Read the model definition and answer for the solid it produces. Units are mm, in the model's axes. A direction names the side the tool comes from. Coordinates: 2 decimals unless noted, no trailing zeros. Order: outer loops, then holes, each group sorted by start corner. A loop starts at its lowest first (then second) coordinate and runs counter-clockwise, first axis right, second up. Notation, with made-up numbers: (72, 72.25) -> (87, 72.25) arc R19 ccw to (87, 103.25) -> close; hole circle Ø3 at (10, -32.5). An arc over 180 degrees is marked (long way). Answer as a JSON object with one key per item and string values. Group by question number.
1) Section C-C on x = 11 is taken. Determine the outline of the cut face in (y, z) (3 decimals).
2) A tool of negligible diameter and unlimited length cuts with its end or side. For faces 1 (the flat face through (-16.036, 26.611, 7.55)), 2 (the flat face through (10.173, -4.366, 4.696)), 3 (the cylindrical face through (-31.266, 33.461, 4.696)), from which of +Z, -Z, +X, -X, +Y, -Y can it reach the whole face along a straight path? Write none if from no direction.
3) Consider L1, parallel to Z at x = 0, y = 57.7 (3 decimals); L2, parallel to Y at x = 19.5, z = 6.25; L3, parallel to Y at x = 1.5, z = 3.25. Determine where each line is inside the solid, lowest interval first.
4) Given pin 1 (3 mm diameter, centred on x = -0.5, z = 5, fed in from -Y); pin 2 (3 mm diameter, centred on x = 12.5, z = 8.5, fed in from -Y); pin 3 (5 mm diameter, centred on x = 0, y = 13.5, fed in from +Z) (3 decimals), each flat-ended and moving along its own axis, determine where each tip first touches the part or whether it passes through.
5) Determine the mould class of faces 4 (the cylindrical face through (-31.23, -0.04, 4.7)), 5 (the cylindrical face through (6.45, 23.53, 1.25)), 6 (the flat face through (17.07, 54.53, 4.7)) for opening direction X: released by +X, released by -X, zero draft, split by the parting line, or undercut.
6) Section A-A on x = -9.5 is taken. Determine the outline of the cut face in (y, z) (3 decimals), and give its area (3 significant figures).
7) Section B-B on y = 53.5 is taken. Determine the outline of the cut face in (x, z) (1 decimal), and give its area (3 significant figures).
8) Section D-D on y = 7 is taken. Determine the outline of the cut face in (x, z) (3 decimals), and give its area (3 significant figures).
from build123d import *

# Parameters (mm, degrees)
F0_R        = 3.1496
F0_R_2      = 16.51
F1_DEPTH    = 9.525
F0_R_3      = 13.97
F2_DEPTH    = 2.54
F4_DEPTH    = 8.636
F5_T1_DEPTH = 2.54
F5_T3_DEPTH = 2.54
F5_T5_DEPTH = 2.54
F5_T7_DEPTH = 2.54
F5_T9_DEPTH = 2.54
F6_R        = 1.5875
F9_DEPTH    = 5.08
F7_R        = 1.5875
F10_DEPTH   = 20.32
F8_R        = 1.5875
F11_DEPTH   = 20.32
F13_DEPTH   = 2.54


# Not quite as in the source:
# - a fillet or chamfer that OpenCascade refuses, or shapes differently, is made with other operations: its cross-section is extruded or revolved along the edge and cut away or added
# - a feature names something its author has since deleted; it is built from what else it names


with BuildPart() as f1:
    # F0 (on Top) → F1 (new body)
    with BuildSketch(Plane.XY):
        with BuildLine():
            ThreePointArc((6.8331158271, 57.7357942584), (0, 58.780934), (-6.8331158271, 57.7357942584))
            Line((-6.8331158271, 57.7357942584), (-27.0242026981, 51.4112964789))
            ThreePointArc((-27.0242026981, 51.4112964789), (-30.2435047856, 49.1112435687), (-31.4761149683, 45.3516130738))
            Line((-31.4761149683, 45.3516130738), (-31.4761149683, 35.0824113719))
            ThreePointArc((-31.4761149683, 35.0824113719), (-31.2597439653, 33.4389104355), (-30.6253762824, 31.9074113719))
            Line((-30.6253762824, 31.9074113719), (-23.4250291837, 19.436044365))
            ThreePointArc((-23.4250291837, 19.436044365), (-22.5749179632, 16.1717783736), (-23.516459851, 12.9327012793))
            Line((-23.516459851, 12.9327012793), (-30.5339456151, 1.5308194413))
            ThreePointArc((-30.5339456151, 1.5308194413), (-31.2360341416, -0.0679607815), (-31.4761149683, -1.7975236443))
            Line((-31.4761149683, -1.7975236443), (-31.4761149683, -7.259066))
            ThreePointArc((-31.4761149683, -7.259066), (-25.5004563551, -15.4606163037), (-15.8622501042, -12.2858874155))
            Line((-15.8622501042, -12.2858874155), (-4.6415514186, 3.3342503548))
            ThreePointArc((-4.6415514186, 3.3342503548), (0, 5.715), (4.6415514186, 3.3342503548))
            Line((4.6415514186, 3.3342503548), (15.8622501042, -12.2858874155))
            ThreePointArc((15.8622501042, -12.2858874155), (25.5004563551, -15.4606163037), (31.4761149683, -7.259066))
            Line((31.4761149683, -7.259066), (31.4761149683, -1.7975236443))
            ThreePointArc((31.4761149683, -1.7975236443), (31.2360341416, -0.0679607815), (30.5339456151, 1.5308194413))
            Line((30.5339456151, 1.5308194413), (23.516459851, 12.9327012793))
            ThreePointArc((23.516459851, 12.9327012793), (22.5749179632, 16.1717783736), (23.4250291837, 19.436044365))
            Line((23.4250291837, 19.436044365), (30.6253762824, 31.9074113719))
            ThreePointArc((30.6253762824, 31.9074113719), (31.2597439653, 33.4389104355), (31.4761149683, 35.0824113719))
            Line((31.4761149683, 35.0824113719), (31.4761149683, 45.3516130738))
            ThreePointArc((31.4761149683, 45.3516130738), (30.2435047856, 49.1112435687), (27.0242026981, 51.4112964789))
            Line((27.0242026981, 51.4112964789), (6.8331158271, 57.7357942584))
        make_face()
        with Locations((-22.86, -7.259066)):
            Circle(F0_R, mode=Mode.SUBTRACT)
        with Locations((22.86, -7.259066)):
            Circle(F0_R, mode=Mode.SUBTRACT)
        with Locations((-22.86, 33.380934)):
            Circle(F0_R, mode=Mode.SUBTRACT)
        with Locations((0, 35.920934)):
            Circle(F0_R_2, mode=Mode.SUBTRACT)
        with Locations((22.86, 33.380934)):
            Circle(F0_R, mode=Mode.SUBTRACT)
    extrude(amount=F1_DEPTH)

    # F0 (on Top) → F2 (join)
    with BuildSketch(Plane.XY):
        with Locations((0, 35.920934)):
            Circle(F0_R_2)
        with Locations((0, 35.920934)):
            Circle(F0_R_3, mode=Mode.SUBTRACT)
    extrude(amount=F2_DEPTH)

    # F3 (on face) → F4 (cut)
    with BuildSketch(Plane.XY.offset(9.525)):
        Polygon((17.6453415423, 29.39956552), (14.4703415423, 23.900304206), (16.6700460679, 22.630304206), (19.8450460679, 28.12956552), align=None)
        Polygon((-3.175, 57.002932274), (-3.175, 54.462932274), (0, 54.462932274), (3.175, 54.462932274), (3.175, 57.002932274), align=None)
        Polygon((-14.4703415423, 23.900304206), (-17.6453415423, 29.39956552), (-19.8450460679, 28.12956552), (-16.6700460679, 22.630304206), align=None)
    extrude(amount=-F4_DEPTH, mode=Mode.SUBTRACT)

    # F5: chamfer of 3.175 x 5.499261314 on 6 edges, made by hand

    # F5_s2 → F5_t1 (join)
    with BuildSketch(Plane(origin=(-0.5036208564, -0.290765637, 0), x_dir=(0, 0, 1), z_dir=(-0.8660254038, -0.5, 0))):
        Polygon((4.064, 34.2834413717), (0.889, 28.7841800576), (0.889, 34.2834413717), align=None)
    extrude(amount=F5_T1_DEPTH)

    # F5_s4 → F5_t3 (join)
    with BuildSketch(Plane(origin=(-2.703325382, -1.560765637, 0), x_dir=(0, 0, 1), z_dir=(0.8660254038, 0.5, 0))):
        Polygon((4.064, -27.9334413717), (0.889, -33.4327026857), (0.889, -27.9334413717), align=None)
    extrude(amount=F5_T3_DEPTH)

    # F5_s6 → F5_t5 (join)
    with BuildSketch(Plane.XZ.offset(-57.002932274)):
        Polygon((-3.175, 4.064), (2.324261314, 0.889), (-3.175, 0.889), align=None)
        Polygon((3.175, 4.064), (-2.324261314, 0.889), (3.175, 0.889), align=None)
    extrude(amount=F5_T5_DEPTH)

    # F5_s8 → F5_t7 (join)
    with BuildSketch(Plane(origin=(2.703325382, -1.560765637, 0), x_dir=(0, 0, 1), z_dir=(-0.8660254038, 0.5, 0))):
        Polygon((4.064, 34.2834413717), (0.889, 28.7841800576), (0.889, 34.2834413717), align=None)
    extrude(amount=F5_T7_DEPTH)

    # F5_s10 → F5_t9 (join)
    with BuildSketch(Plane(origin=(0.5036208564, -0.290765637, 0), x_dir=(0, 0, 1), z_dir=(0.8660254038, -0.5, 0))):
        Polygon((4.064, -27.9334413717), (0.889, -33.4327026857), (0.889, -27.9334413717), align=None)
    extrude(amount=F5_T9_DEPTH)

    # F6 (on face) → F9 (cut, symmetric)
    with BuildSketch(Plane.XZ.offset(-57.002932274)):
        with Locations((0, 5.8970871047)):
            Circle(F6_R)
    extrude(amount=F9_DEPTH, both=True, mode=Mode.SUBTRACT)

    # F7 (on face) → F10 (cut, symmetric)
    with BuildSketch(Plane(origin=(-2.703325382, -1.560765637, 0), x_dir=(-0.5, 0.8660254038, 0), z_dir=(0.8660254038, 0.5, 0))):
        with Locations((31.0334954411, 5.6098689985)):
            Circle(F7_R)
    extrude(amount=F10_DEPTH, both=True, mode=Mode.SUBTRACT)

    # F8 (on face) → F11 (cut, symmetric)
    with BuildSketch(Plane(origin=(2.703325382, -1.560765637, 0), x_dir=(-0.5, -0.8660254038, 0), z_dir=(-0.8660254038, 0.5, 0))):
        with Locations((-31.1158668548, 5.8928)):
            Circle(F8_R)
    extrude(amount=F11_DEPTH, both=True, mode=Mode.SUBTRACT)

    # F12 (on face) → F13 (cut)
    with BuildSketch(Plane.XY.offset(9.525)):
        Polygon((3.2258, 11.1985175016), (3.2258, 14.9233504984), (0, 16.7857669967), (-3.2258, 14.9233504984), (-3.2258, 11.1985175016), (0, 9.3361010033), align=None)
    extrude(amount=-F13_DEPTH, mode=Mode.SUBTRACT)


with BuildPart() as f14_1:
    # F14: copy of F1
    add(f1.part)


solid = f1.part
Worked answers:
{
 "1": {"outline": "(-5.517, 0) -> (27.309, 0) -> (27.309, 2.54) -> (23.609, 2.54) -> (23.609, 9.525) -> (-5.517, 9.525) -> close; (44.533, 0) -> (56.431, 0) -> (56.431, 9.525) -> (48.233, 9.525) -> (48.233, 2.54) -> (44.533, 2.54) -> close"},
 "2": {"face 1": "+Z", "face 2": "+Z, -Z, -Y", "face 3": "+Z, -Z, -X"},
 "3": {"L1": "z = 0 to 4.31, 7.485 to 9.525", "L2": "y = -15.19 to 22.89, 26.46 to 27.53, 28.33 to 53.77", "L3": "y = 5.51 to 19.48, 52.36 to 54.46, 57 to 58.73"},
 "4": {"pin 1": "stops at y = 5.35", "pin 2": "stops at y = -9.69", "pin 3": "stops at z = 6.985"},
 "5": {"face 4": "released by -X", "face 5": "undercut", "face 6": "released by +X"},
 "6": {"outline": "(-3.429, 0) -> (25.678, 0) -> (25.678, 2.54) -> (22.418, 2.54) -> (22.418, 9.525) -> (-3.429, 9.525) -> close; (46.164, 0) -> (56.9, 0) -> (56.9, 9.525) -> (49.424, 9.525) -> (49.424, 2.54) -> (46.164, 2.54) -> close", "area": "334 mm²"},
 "7": {"outline": "(-20.4, 0) -> (20.4, 0) -> (20.4, 9.5) -> (-20.4, 9.5) -> close; hole circle Ø3.2 at (0, 5.9)", "area": "380 mm²"},
 "8": {"outline": "(-27.168, 0) -> (27.168, 0) -> (27.168, 9.525) -> (-27.168, 9.525) -> close", "area": "518 mm²"}
}
